Check sheet for the modelled part. Datum: model origin and axes. Units: mm. A direction names the side the tool comes from. Coordinates: 2 decimals unless noted, no trailing zeros. Write each loop counter-clockwise with the first axis right and the second up, starting at its lowest first coordinate (ties: lowest second). Pieces come first, ordered by that corner, then holes. Notation, with made-up numbers: M -7,23.25 L 18,23.25 A33 ccw 18,57.25 Z; hole C -9,-29 d3. An arc over 180 degrees is marked long. Answer as CSV lines item,"result".
from build123d import *

# Parameters (mm, degrees)
EXTRUDE_1_DEPTH     = 55
CUT_EXTRUDE_1_DEPTH = 7
CUT_EXTRUDE_2_DEPTH = 12
SKETCH_5_R          = 1.9
CUT_EXTRUDE_3_DEPTH = 35
SKETCH_6_W          = 0.8
SKETCH_6_H          = 6.8
CUT_EXTRUDE_4_DEPTH = 7
SKETCH_7_W          = 0.8
SKETCH_7_H          = 6.8
CUT_EXTRUDE_5_DEPTH = 12


with BuildPart() as part:
    # 草图2 → 凸台-拉伸1 (new body)
    with BuildSketch(Plane(origin=(0, 0, 0), x_dir=(1, 0, 0), z_dir=(0, 1, 0))):
        Polygon((3.92598183, 0), (1.962990915, 3.4), (-1.962990915, 3.4), (-3.92598183, 0), (-1.962990915, -3.4), (1.962990915, -3.4), align=None)
    extrude(amount=EXTRUDE_1_DEPTH)

    # 草图3 → 切除-拉伸1 (cut)
    with BuildSketch(Plane(origin=(0, 55, 0), x_dir=(1, 0, 0), z_dir=(0, 1, 0))):
        with BuildLine():
            Line((1.161895004, 1.1), (-1.161895004, 1.1))
            ThreePointArc((-1.161895004, 1.1), (-0.592016889, -1.48644408), (1.6, 0))
            ThreePointArc((1.6, 0), (1.48644408, 0.592016889), (1.161895004, 1.1))
        make_face()
    extrude(amount=-CUT_EXTRUDE_1_DEPTH, mode=Mode.SUBTRACT)

    # 草图4 → 切除-拉伸2 (cut)
    with BuildSketch(Plane.XZ):
        Polygon((-1.5011107, -2.6), (1.5011107, -2.6), (3.0022214, 0), (1.5011107, 2.6), (-1.5011107, 2.6), (-3.0022214, 0), align=None)
    extrude(amount=-CUT_EXTRUDE_2_DEPTH, mode=Mode.SUBTRACT)

    # 草图5 → 切除-拉伸3 (cut)
    with BuildSketch(Plane.XZ.offset(-12)):
        with Locations(Location((0, 0, 0), (0, 0, 270))):
            Circle(SKETCH_5_R)
    extrude(amount=-CUT_EXTRUDE_3_DEPTH, mode=Mode.SUBTRACT)

    # 草图6 → 切除-拉伸4 (cut)
    with BuildSketch(Plane(origin=(0, 55, 0), x_dir=(1, 0, 0), z_dir=(0, 1, 0))):
        Rectangle(SKETCH_6_W, SKETCH_6_H)
    extrude(amount=-CUT_EXTRUDE_4_DEPTH, mode=Mode.SUBTRACT)

    # 草图7 → 切除-拉伸5 (cut)
    with BuildSketch(Plane.XZ):
        Rectangle(SKETCH_7_W, SKETCH_7_H)
    extrude(amount=-CUT_EXTRUDE_5_DEPTH, mode=Mode.SUBTRACT)


solid = part.part
1) Mould release check, pull along X, two halves, no side actions. Record for faces 1 (the face through (-0.4, 52, -2)), 2 (the face through (-3, 0, -1)), 3 (the face through (2.931, 27.115, 1.724)): pulls with the +X half, pulls with the -X half, needs draft (parallel to the pull), parting line crosses it, or undercut.
Answer key:
face 1,"undercut"
face 2,"needs draft"
face 3,"pulls with the +X half"
2) Section check A-A, the plane y = 29. Record the boundary of the cut face in (x, z), plus the area to 3 significant figures.
Answer key:
outline,"M -3.93,0 L -1.96,-3.4 L 1.96,-3.4 L 3.93,0 L 1.96,3.4 L -1.96,3.4 Z; hole C 0,0 d3.8"
area,"28.7 mm2"
3) Depth check by flat-ended pin: P1, Ø0.9, axis at y = 8, z = -3, coming from the -X side; P2, Ø2, axis at y = 50.5, z = 2.5, coming from the -X side; P3, Ø1.5, axis at x = -3, y = 45, coming from the +Z side. Enter the tip coordinate at first touch or a pass-through.
Answer key:
P1,"stops at x = -2.45"
P2,"stops at x = -3.06"
P3,"stops at z = 2.9"
4) Thickness scan on line 1 along X through (y, z) = (32, 0); line 2 along Z through (x, y) = (-1.5, 37); line 3 along Z through (x, y) = (3, 30). Record the ranges inside material, lowest first.
Answer key:
line 1,"x = -3.93 to -1.9, 1.9 to 3.93"
line 2,"z = -3.4 to -1.17, 1.17 to 3.4"
line 3,"z = -1.6 to 1.6"
5) Tool access check on faces 4 (the face through (2, 55, 0)), 5 (the face through (-0.728, 29.255, -1.755)), 6 (the face through (-1.544, 51.549, 0.42)), 7 (the face through (0.4, 52, 2)). Record the directions out of +Z, -Z, +X, -X, +Y, -Y that give a thin tool (end or side, any length) a straight path to the whole face; none if there is none.
Answer key:
face 4,"+Z, -Z, +X, -X, +Y"
face 5,"-Y"
face 6,"+Y"
face 7,"+Z, -Z, +Y"
6) Section check B-B, the plane z = -0.5. Record the boundary of the cut face in (x, y).
Answer key:
outline,"M -3.64,0 L -2.71,0 L -2.71,12 L -1.83,12 L -1.83,47 L 1.83,47 L 1.83,12 L 2.71,12 L 2.71,0 L 3.64,0 L 3.64,55 L 1.52,55 L 1.52,48 L -1.52,48 L -1.52,55 L -3.64,55 Z"
